Read the model definition and answer for the solid it produces. Units are mm, in the model's axes. Face numbers are marked on the shaded views. A direction names the side the tool comes from. Coordinates: 2 decimals unless noted, no trailing zeros. Write each loop counter-clockwise with the first axis right and the second up, starting at its lowest first coordinate (ties: lowest second). Pieces come first, ordered by that corner, then holes.
(1) Section C-C on y = 0 is taken. Write down the section's boundary in (x, z).
(2) Find the intervals of material crossed by probe 1 along X at (y, z) = (-3.5, 40); probe 2 along Z at (x, y) = (0, 0); probe 3 along Z at (x, y) = (0, -5.75), in increasing order.
(3) Section B-B on x = 0 is taken. Write down the section's boundary in (y, z).
(4) Given pin 1 (1.5 mm diameter, centred on x = 6, y = 3.5, fed in from +Z); pin 2 (2 mm diameter, centred on x = -3.5, y = 5.5, fed in from -Z), each flat-ended and moving along its own axis, determine where each tip first touches the part or whether it passes through.
(5) Section A-A on z = 40 is taken. Write down the section's boundary in (x, y).
(6) Which of the six approach directions +Z, -Z, +X, -X, +Y, -Y give full straight-line access (tool end or side, diameter ignored) to the marked faces 1, 2 and 3?
(7) The mould has two halves that part along X. Classify the marked faces 4, 5 and 6: +X half, -X half, draft (parallel to the pull), parting line (faces both ways), or undercut.
(8) Section D-D on y = -8 is taken. Write down the section's boundary in (x, z).
Autodesk Inventor part; units mm, degrees
ref_plane "Work Plane1" through (0, 0, 40) normal (0, 0, 1) x (1, 0, 0)
ref_plane "Work Plane2" through (-8, 10, 0) normal (0, 1, 0) x (1, 0, 0)
ref_plane "YZ Plane" through (0, 0, 0) normal (1, 0, 0) x (0, 1, 0)
sketch "Sketch1" plane through (0, 0, 0) normal (0, 0, 1) x (1, 0, 0)
  line L0 (-10, 10) -> (10, 10)
  line L1 (10, 10) -> (10, -10)
  line L2 (10, -10) -> (-10, -10)
  line L3 (-10, -10) -> (-10, 10)
  line L4 (-10, 10) -> (10, -10) construction
  line L5 (10, 10) -> (-10, -10) construction
  point P0 (0, 0)
  dimension "d0" = 20
  dimension "d1" = 20
extrude "Extrusion1" add sketch "Sketch1" along normal blind 80
sketch "Sketch2" plane through (0, 0, 80) normal (0, 0, 1) x (1, 0, 0)
  circle A0 centre (0, 0) radius 4.75
  dimension "d4" = 9.5
extrude "Extrusion2" add sketch "Sketch2" along normal blind 10
ref_plane "Work Plane1" through (0, 0, 40) normal (0, 0, 1) x (1, 0, 0)
mirror "Mirror1" about plane through (0, 0, 40) normal (0, 0, 1) of "Extrusion2"
ref_plane "Work Plane2" through (-8, 10, 0) normal (0, 1, 0) x (1, 0, 0)
sketch "Sketch3" plane through (-8, 10, 0) normal (0, 1, 0) x (1, 0, 0)
  line L0 (-2, -80) -> (-2, 0)
  line L1 (-2, -40) -> (18, -40)
  line L2 (18, 0) -> (18, -80)
  circle A0 centre (8, -40) radius 5.5
  point P0 (8, 0)
  dimension "d8" = 11
extrude "Extrusion3" cut sketch "Sketch3" against normal through all
properties part number "FP V2 Arm Connector"
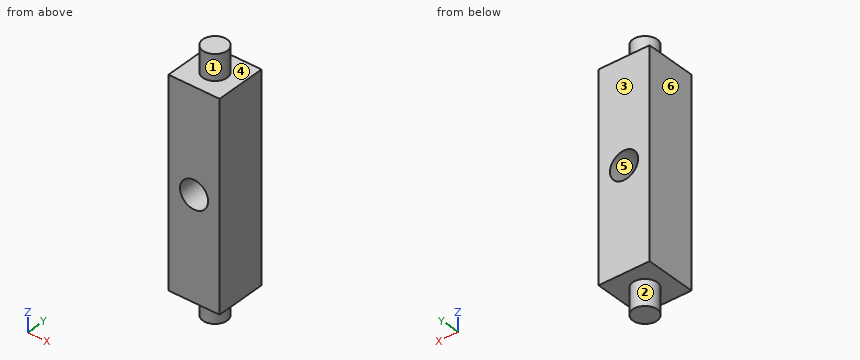
Response:
1. outline: (-10, 0) - (-4.75, 0) - (-4.75, -10) - (4.75, -10) - (4.75, 0) - (10, 0) - (10, 80) - (4.75, 80) - (4.75, 90) - (-4.75, 90) - (-4.75, 80) - (-10, 80) - close; hole circle Ø11 at (0, 40)
2. probe 1: x = -10 to -5.5, 5.5 to 10
2. probe 2: z = -10 to 34.5, 45.5 to 90
2. probe 3: z = 0 to 34.5, 45.5 to 80
3. outline: (-10, 0) - (-4.75, 0) - (-4.75, -10) - (4.75, -10) - (4.75, 0) - (10, 0) - (10, 34.5) - (-10, 34.5) - close; (-10, 45.5) - (10, 45.5) - (10, 80) - (4.75, 80) - (4.75, 90) - (-4.75, 90) - (-4.75, 80) - (-10, 80) - close
4. pin 1: stops at z = 80
4. pin 2: stops at z = 0
5. outline: (-10, -10) - (-5.5, -10) - (-5.5, 10) - (-10, 10) - close; (5.5, -10) - (10, -10) - (10, 10) - (5.5, 10) - close
6. face 1: +Z
6. face 2: -Z
6. face 3: +Z, -Z, +X, -X, +Y
7. face 4: draft
7. face 5: undercut
7. face 6: -X half
8. outline: (-10, 0) - (10, 0) - (10, 80) - (-10, 80) - close; hole circle Ø11 at (0, 40)
